Design review of the part built by this model. Coordinates are the model's own, in mm. A direction names the side the tool comes from. Give positions to 0.01 mm unless a question says otherwise; leave off trailing zeros. Order: outer loops, then holes, each group sorted by start corner. A loop starts at its lowest first (then second) coordinate and runs counter-clockwise, first axis right, second up. Notation, with made-up numbers: M -30,26 L 7,26 A21 ccw 7,48 Z; hole C -26.75,84 d3. An arc over 180 degrees is marked long. Answer as a JSON object with one key per item and string values.
from build123d import *

# Parameters (mm, degrees)
BOSS_EXTRUDE1_DEPTH = 30
SKETCH2_W           = 14.98
SKETCH2_H           = 14.98
BOSS_EXTRUDE2_DEPTH = 10
SKETCH3_W           = 14.98
SKETCH3_H           = 14.98
BOSS_EXTRUDE3_DEPTH = 40
FILLET1_R           = 5


with BuildPart() as part:
    # Sketch1 → Boss-Extrude1 (new body)
    with BuildSketch(Plane.XY):
        Polygon((0, 0), (-30, 0), (-112.5, 235), (-112.5, 265), (-82.5, 265), (0, 30), align=None)
    extrude(amount=BOSS_EXTRUDE1_DEPTH)

    # Sketch2 → Boss-Extrude2 (add)
    with BuildSketch(Plane.ZY.offset(112.5)):
        with Locations((15, 250)):
            Rectangle(SKETCH2_W, SKETCH2_H)
    extrude(amount=BOSS_EXTRUDE2_DEPTH)

    # Sketch3 → Boss-Extrude3 (add)
    with BuildSketch(Plane.XZ):
        with Locations((-15, 15)):
            Rectangle(SKETCH3_W, SKETCH3_H)
    extrude(amount=BOSS_EXTRUDE3_DEPTH)

    # Fillet1
    fillet1_edges = [part.edges().sort_by_distance(p)[0] for p in [
        (-82.5, 265, 15),
        (0, 30, 15),
    ]]
    fillet(fillet1_edges, radius=FILLET1_R)


solid = part.part
(1) We need section B-B (x = -14). Write out the cut boundary in (y, z), plus the area to 3 significant figures.
Checked values:
{"outline": "M -40,7.51 L 0,7.51 L 0,0 L 69.88,0 L 69.88,30 L 0,30 L 0,22.49 L -40,22.49 Z", "area": "2,700 mm^2"}
(2) Tool access review of faces 1 (the flat face through (-15, -20, 22.49)), 2 (the flat face through (-7.51, -20, 15)), 3 (the flat face through (-117, 242.51, 15)), 4 (the flat face through (-117, 250, 22.49)): name each direction out of +Z, -Z, +X, -X, +Y, -Y from which nothing blocks a thin tool from reaching the whole face with its end or side.
Checked values:
{"face 1": "+Z, +X, -X, -Y", "face 2": "+Z, -Z, +X, -Y", "face 3": "+Z, -Z, -X, -Y", "face 4": "+Z, -X, +Y, -Y"}
(3) We need section C-C (y = 7). Write out the cut boundary in (x, z), plus the area to 3 significant figures.
Checked values:
{"outline": "M -32.46,0 L 0,0 L 0,30 L -32.46,30 Z", "area": "974 mm^2"}
(4) We need section A-A (z = 15.25). Write out the cut boundary in (x, y), plus the area to 3 significant figures.
Checked values:
{"outline": "M -122.5,242.51 L -112.5,242.51 L -112.5,235 L -30,0 L -22.49,0 L -22.49,-40 L -7.51,-40 L -7.51,0 L 0,0 L 0,29.15 A5 ccw -0.28,30.8 L -81.33,261.66 A5 ccw -86.04,265 L -112.5,265 L -112.5,257.49 L -122.5,257.49 Z", "area": "11,200 mm^2"}
(5) We need section D-D (x = -39.5). Write out the cut boundary in (y, z), plus the area to 3 significant figures.
Checked values:
{"outline": "M 27.06,0 L 142.52,0 L 142.52,30 L 27.06,30 Z", "area": "3,460 mm^2"}
(6) Insertion check: pin 1 (10 mm diameter, centred on x = -55.5, y = 210, fed in from -Z); pin 2 (4.5 mm diameter, centred on y = -22, z = 13, fed in from -X); pin 3 (8 mm diameter, centred on y = 204, z = 17, fed in from +X); pin 4 (1.5 mm diameter, centred on y = 162.5, z = 24, fed in from +X). Each pin has a flat end and moves straight along its axis. Give the tip position at first contact, or say it passes through.
Checked values:
{"pin 1": "passes through", "pin 2": "stops at x = -22.49", "pin 3": "stops at x = -59.68", "pin 4": "stops at x = -46.25"}
(7) To check wall thickness, follow L1, parallel to X at y = 111.5, z = 12.75; L2, parallel to Z at x = -8.5, y = -20.5; L3, parallel to X at y = 235.5, z = 12.5. State the ranges of each line that lie inside material, in increasing order. Write a range as from..to.
Checked values:
{"L1": "x = -69.14..-28.61", "L2": "z = 7.51..22.49", "L3": "x = -112.5..-72.14"}
